from build123d import *

# Parameters (mm, degrees)
F1_DEPTH = 35
F1_TAPER = -30
F2_DEPTH = 60
F2_TAPER = 30


with BuildPart() as f1:
    # F0 (on Top) → F1 (new body)
    with BuildSketch(Plane.XY):
        Polygon((-25.7642557626, -14.875), (0, -29.75), (25.7642557626, -14.875), (25.7642557626, 14.875), (0, 29.75), (-25.7642557626, 14.875), align=None)
    extrude(amount=F1_DEPTH, taper=F1_TAPER)

    # F1_face (on face) → F2 (join)
    with BuildSketch(Plane.XY.offset(35)):
        Polygon((-45.9715151842, -26.5416666667), (0, -53.0833333333), (45.9715151842, -26.5416666667), (45.9715151842, 26.5416666667), (0, 53.0833333333), (-45.9715151842, 26.5416666667), align=None)
    extrude(amount=F2_DEPTH, taper=F2_TAPER)


solid = f1.part
Build history of the part. All positions in model axes, mm. Round coordinates to 2 decimals unless told otherwise and drop trailing zeros. Write each loop counter-clockwise with the first axis right and the second up, starting at its lowest first coordinate (ties: lowest second). Pieces come first, ordered by that corner, then holes. Notation, with made-up numbers: M -27.75,29.25 L -6.75,29.25 A26 cw -6.75,64.25 Z; hole C 0.5,-2 d7. An arc over 180 degrees is marked long. Use CSV: the item, a comma, the result in double quotes.
1. Saw through at B-B (z = 54.5). Give the cut face in (x, y), plus the area to 3 significant figures.
Reply:
outline,"M -34.71,-20.04 L 0,-40.08 L 34.71,-20.04 L 34.71,20.04 L 0,40.08 L -34.71,20.04 Z"
area,"4,170 mm²"
2. Wall check: probe 1 along Y at (x, z) = (-27.5, 29); probe 2 along Y at (x, z) = (18, 12); probe 3 along Z at (x, y) = (-21, 36). Give the ranges that are in metal, low to high. Write a range as from..to.
Reply:
probe 1,"y = -33.21..33.21"
probe 2,"y = -27.36..27.36"
probe 3,"z = 27.56..42.44"
3. Saw through at A-A (z = 69.5). Give the cut face in (x, y), plus the area to 3 significant figures.
Reply:
outline,"M -26.05,-15.04 L 0,-30.08 L 26.05,-15.04 L 26.05,15.04 L 0,30.08 L -26.05,15.04 Z"
area,"2,350 mm²"
4. Flat gauge pins, fed straight in: pin 1 (6 mm diameter, centred on x = -24.5, y = -12.5, fed in from +Z); pin 2 (2 mm diameter, centred on y = -7.5, z = 52, fed in from +X); pin 3 (2 mm diameter, centred on x = 34, y = -26.5, fed in from -Z). Where does each tip first touch, or does it go through?
Reply:
pin 1,"stops at z = 77.38"
pin 2,"stops at x = 36.73"
pin 3,"stops at z = 22.84"
